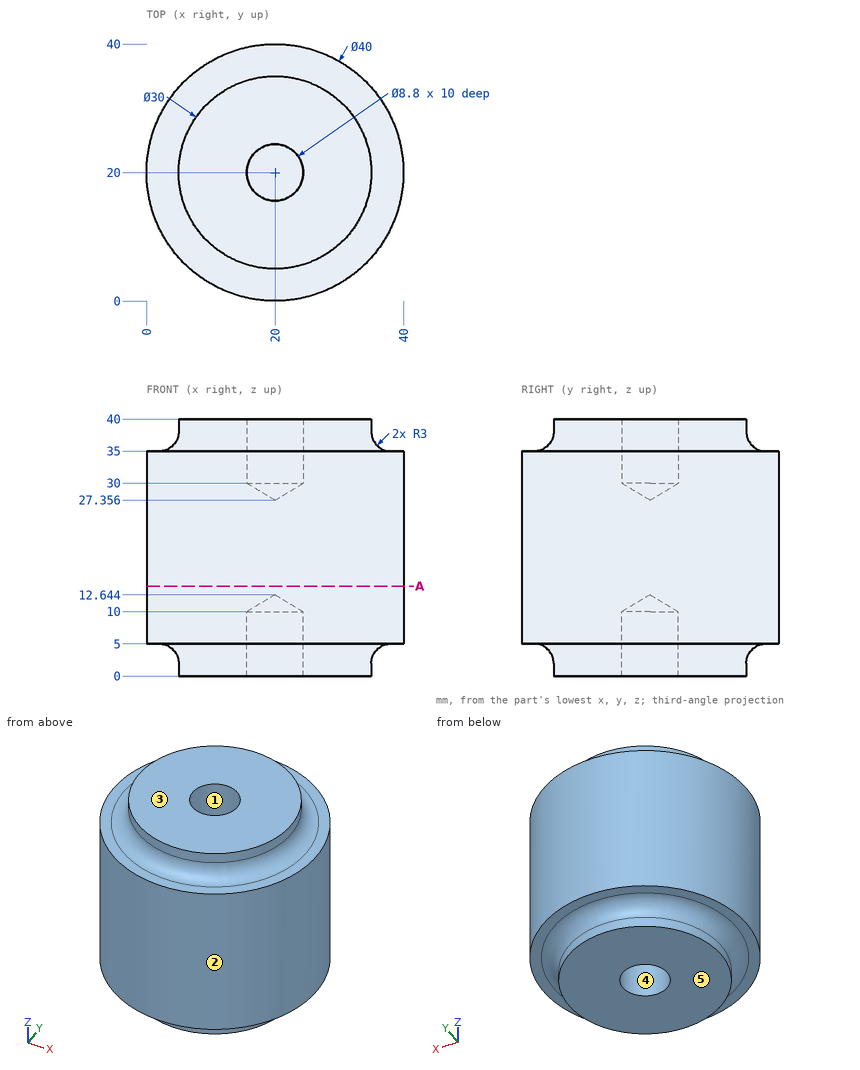
Source: three-view drawing plus pictorial views. Frame: mm from the lowest corner of the part. A direction names the side the tool comes from. Round coordinates to 2 decimals unless told otherwise and drop trailing zeros. Order: outer loops, then holes, each group sorted by start corner. A loop starts at its lowest first (then second) coordinate and runs counter-clockwise, first axis right, second up. Notation, with made-up numbers: (24.25, 80.25) -> (68.25, 80.25) arc R19 ccw to (68.25, 103.25) -> close; hole circle Ø2 at (74.25, 22.25). An arc over 180 degrees is marked (long way). Use one line per item in the form item = value. Start each with the question number.
1. Line query: probe 1 along Y at (x, z) = (20, 7); probe 2 along Z at (x, y) = (9.5, 3.5); probe 3 along Y at (x, z) = (21.5, 29) (1 decimal). Output: solid intervals per line, ascending.
2. Cut plane A-A (z = 14). Return the cut outline in (x, y).
3. Reachability of the marked faces 4 and 5 from +Z, -Z, +X, -X, +Y, -Y: full face, straight path, thin tool, end or side. Return the list, or none.
4. Pin query (flat end, axial travel): pin 1 Ø5 at (y, z) = (13, 19) entering from +X; pin 2 Ø6 at (x, y) = (7, 34.5) entering from +Z; pin 3 Ø6 at (x, y) = (19.5, 20.5) entering from -Z. Return the tip coordinate at first contact, or that it passes through.
5. Draft query along Y for the marked faces 1, 2 and 3. Return one class per face: pulls with the +Y half, pulls with the -Y half, needs draft (parallel to the pull), parting line crosses it, or undercut.
Solution:
q1.probe_1 = 0 to 15.6, 24.4 to 40
q1.probe_2 = 5 to 35
q1.probe_3 = 0.1 to 17.7, 22.3 to 39.9
q2.outline = circle Ø40 at (20, 20)
q3.face_4 = -Z
q3.face_5 = -Z, +X, -X, +Y, -Y
q4.pin_1 = 39.49
q4.pin_2 = 35.42
q4.pin_3 = 10.42
q5.face_1 = undercut
q5.face_2 = parting line crosses it
q5.face_3 = needs draft
